Here's how the part is built. I have some questions about the finished solid (model axes, mm). A direction names the side the tool comes from. Give positions to 0.01 mm unless a question says otherwise; leave off trailing zeros. Loops run counter-clockwise (first coordinate to the right, second up) from the corner with the lowest first, then second, coordinate; pieces in that order, holes last. Notation, with made-up numbers: (81.25, -5.75) - (96.25, -5.75) arc R18 cw to (96.25, 23.25) - close; hole circle Ø4 at (70.5, 89). An arc over 180 degrees is marked (long way). Return JSON: item names as keys, results as strings. Group by question number.
(1) If we mould it in two halves opening along Y, with no side actions, what happens to faces 4 (the flat face through (-24, 15, -66)), 5 (the flat face through (-50, -10, -50)), 6 (the flat face through (72, -5, 7))? For each: released by +Y, released by -Y, zero draft, split by the parting line, or undercut.
(2) If we section it at C-C (y = 4.5): Please give me the cut outline in (x, z), then the cut area to 3 significant figures.
(3) On a 3-axis mill with a long thin cutter (end or side, diameter ignored), from which of +Z, -Z, +X, -X, +Y, -Y can I reach the whole of each face in a straight line? I mean faces 1 (the cylindrical face through (-42.594, 2.325, -55.55)), 2 (the cylindrical face through (-45.636, -12.535, 59.517)), 3 (the flat face through (-42, -5, 59)). Say none if no direction works.
(4) For P1, Ø2, axis at y = 1, z = 43.5, coming from the -X side; P2, Ø2, axis at y = -10.5, z = -22, coming from the -X side; P3, Ø5, axis at x = 71, z = 5, coming from the -Y side; P4, Ø6, axis at x = -43, z = -48, coming from the -Y side, each with a flat end and sliding along its axis, tell me the tip position at first contact or that it passes through.
(5) If we section it at B-B (z = 27): Please give me the cut outline in (x, y).
(6) If we section it at A-A (x = 0): Please give me the cut outline in (y, z).
(7) I need wall thicknesses on probe 1 along X at (y, z) = (-1.25, 2); probe 2 along X at (y, z) = (-11.2, 0); probe 3 along Z at (x, y) = (-23.5, 9.25). Which ranges of each line are inside material? Lowest first, please. Write a range as [from, to].
```python
from build123d import *

# Parameters (mm, degrees)
SKETCH_1_R               = 81
SKETCH_1_R_2             = 70
EXTRUDE_1_DEPTH          = 15
SKETCH_2_W               = 5
SKETCH_2_H               = 2.5
CUT_REVOLVE_1_ANGLE      = 10
PATTERN_CIRCULAR_1_COUNT = 3
SKETCH_3_R               = 75
CUT_EXTRUDE_1_DEPTH      = 5


with BuildPart() as part:
    # 草圖1 → 填料-伸長1 (new, symmetric)
    with BuildSketch(Plane(origin=(0, 0, 0), x_dir=(1, 0, 0), z_dir=(0, 1, 0))):
        with Locations(Location((0, 0, 0), (0, 0, 270))):
            Circle(SKETCH_1_R)
        with Locations(Location((0, 0, 0), (0, 0, 270))):
            Circle(SKETCH_1_R_2, mode=Mode.SUBTRACT)
    extrude(amount=EXTRUDE_1_DEPTH, both=True)

    # 草圖2 → 除料-旋轉1 (revolve, cut)
    with BuildSketch(Plane.XY):
        with Locations((72.498409613, -3.75)):
            Rectangle(SKETCH_2_W, SKETCH_2_H)
    cut_revolve_1 = revolve(axis=Axis((0, 15, 0), (0, -1, 0)), revolution_arc=CUT_REVOLVE_1_ANGLE, mode=Mode.SUBTRACT)

    # 環狀複製排列1: 除料-旋轉1 ×3 about axis
    pattern_circular_1_axis = Axis((0, 0, 0), (0, 1, 0))
    for i in range(1, PATTERN_CIRCULAR_1_COUNT):
        add(cut_revolve_1.rotate(pattern_circular_1_axis, i * 360 / PATTERN_CIRCULAR_1_COUNT), mode=Mode.SUBTRACT)

    # 草圖3 → 除料-伸長1 (cut)
    with BuildSketch(Plane.XZ.offset(15)):
        with Locations(Location((0, 0, 0), (0, 0, 270))):
            Circle(SKETCH_3_R)
    extrude(amount=-CUT_EXTRUDE_1_DEPTH, mode=Mode.SUBTRACT)


solid = part.part
```
Values:
{
 "1": {"face 4": "released by +Y", "face 5": "released by -Y", "face 6": "undercut"},
 "2": {"outline": "circle Ø162 at (0, 0); hole circle Ø140 at (0, 0)", "area": "5,220 mm2"},
 "3": {"face 1": "+Y, -Y", "face 2": "-Y", "face 3": "none"},
 "4": {"P1": "x = -68.95", "P2": "x = -78.23", "P3": "y = -10", "P4": "through"},
 "5": {"outline": "(-76.37, -15) - (-69.97, -15) - (-69.97, -10) - (-64.58, -10) - (-64.58, 15) - (-76.37, 15) - close; (64.58, -10) - (69.97, -10) - (69.97, -15) - (76.37, -15) - (76.37, 15) - (64.58, 15) - close"},
 "6": {"outline": "(-15, -81) - (15, -81) - (15, -70) - (-10, -70) - (-10, -75) - (-15, -75) - close; (-15, 75) - (-10, 75) - (-10, 70) - (15, 70) - (15, 81) - (-15, 81) - close"},
 "7": {"probe 1": "[-80.98, -69.97], [69.97, 80.98]", "probe 2": "[-81, -75], [75, 81]", "probe 3": "[-77.52, -65.94], [65.94, 77.52]"}
}
